from build123d import *

# Parameters (mm, degrees)
SKETCH1_R           = 10.75
SKETCH1_R_2         = 9.75
BOSS_EXTRUDE1_DEPTH = 1
SKETCH2_R           = 10.75
SKETCH2_R_2         = 9.75
BOSS_EXTRUDE2_DEPTH = 3.5
SKETCH3_R           = 10.75
BOSS_EXTRUDE3_DEPTH = 1.5
CUT_EXTRUDE1_DEPTH  = 1
BOSS_EXTRUDE4_DEPTH = 6
FILLET1_R           = 1.25
FILLET2_R           = 0.5


with BuildPart() as part:
    # Sketch1 → Boss-Extrude1 (new body)
    with BuildSketch(Plane(origin=(0, 0, 0), x_dir=(1, 0, 0), z_dir=(0, 1, 0))):
        with Locations(Location((0, 0, 0), (0, 0, 270))):
            Circle(SKETCH1_R)
        Circle(SKETCH1_R_2, mode=Mode.SUBTRACT)
        Circle(SKETCH1_R_2)
    extrude(amount=BOSS_EXTRUDE1_DEPTH)

    # Sketch2 → Boss-Extrude2 (add)
    with BuildSketch(Plane(origin=(0, 1, 0), x_dir=(1, 0, 0), z_dir=(0, 1, 0))):
        with Locations(Location((0, 0, 0), (0, 0, 270))):
            Circle(SKETCH2_R)
        with Locations(Location((0, 0, 0), (0, 0, 270))):
            Circle(SKETCH2_R_2, mode=Mode.SUBTRACT)
    extrude(amount=BOSS_EXTRUDE2_DEPTH)

    # Sketch3 → Boss-Extrude3 (add)
    with BuildSketch(Plane(origin=(0, 4.5, 0), x_dir=(1, 0, 0), z_dir=(0, 1, 0))):
        with Locations(Location((0, 0, 0), (0, 0, 270))):
            Circle(SKETCH3_R)
    extrude(amount=BOSS_EXTRUDE3_DEPTH)

    # Sketch4 → Cut-Extrude1 (cut)
    with BuildSketch(Plane(origin=(0, 6, 0), x_dir=(1, 0, 0), z_dir=(0, 1, 0))):
        Polygon((-9.25, -0.5), (-9.75, 0), (-9.25, 0.5), (-0.5, 0.5), (-0.5, 9.25), (0, 9.75), (0.5, 9.25), (0.5, 0.5), (9.25, 0.5), (9.75, 0), (9.25, -0.5), (0.5, -0.5), (0.5, -9.25), (0, -9.75), (-0.5, -9.25), (-0.5, -0.5), align=None)
        with BuildLine():
            ThreePointArc((-1.414213562, -0.5), (-1.5, 0), (-1.414213562, 0.5))
            Line((-1.414213562, 0.5), (-9.25, 0.5))
            Line((-9.25, 0.5), (-9.75, 0))
            Line((-9.75, 0), (-9.25, -0.5))
            Line((-9.25, -0.5), (-1.414213562, -0.5))
        make_face()
        with BuildLine():
            Line((9.25, 0.5), (1.414213562, 0.5))
            ThreePointArc((1.414213562, 0.5), (1.478397839, 0.253652968), (1.5, 0))
            ThreePointArc((1.5, 0), (1.478397839, -0.253652968), (1.414213562, -0.5))
            Line((1.414213562, -0.5), (9.25, -0.5))
            Line((9.25, -0.5), (9.75, 0))
            Line((9.75, 0), (9.25, 0.5))
        make_face()
        with BuildLine():
            Line((-0.5, 9.25), (-0.5, 1.414213562))
            ThreePointArc((-0.5, 1.414213562), (0, 1.5), (0.5, 1.414213562))
            Line((0.5, 1.414213562), (0.5, 9.25))
            Line((0.5, 9.25), (0, 9.75))
            Line((0, 9.75), (-0.5, 9.25))
        make_face()
        with BuildLine():
            ThreePointArc((0.5, -1.414213562), (0, -1.5), (-0.5, -1.414213562))
            Line((-0.5, -1.414213562), (-0.5, -9.25))
            Line((-0.5, -9.25), (0, -9.75))
            Line((0, -9.75), (0.5, -9.25))
            Line((0.5, -9.25), (0.5, -1.414213562))
        make_face()
        with BuildLine():
            Line((-0.5, -0.5), (-1.414213562, -0.5))
            ThreePointArc((-1.414213562, -0.5), (-1.060660172, -1.060660172), (-0.5, -1.414213562))
            Line((-0.5, -1.414213562), (-0.5, -0.5))
        make_face()
        with BuildLine():
            Line((-1.414213562, 0.5), (-0.5, 0.5))
            Line((-0.5, 0.5), (-0.5, 1.414213562))
            ThreePointArc((-0.5, 1.414213562), (-1.060660172, 1.060660172), (-1.414213562, 0.5))
        make_face()
        with BuildLine():
            ThreePointArc((1.414213562, 0.5), (1.060660172, 1.060660172), (0.5, 1.414213562))
            Line((0.5, 1.414213562), (0.5, 0.5))
            Line((0.5, 0.5), (1.414213562, 0.5))
        make_face()
        with BuildLine():
            Line((0.5, -0.5), (0.5, -1.414213562))
            ThreePointArc((0.5, -1.414213562), (1.060660172, -1.060660172), (1.414213562, -0.5))
            Line((1.414213562, -0.5), (0.5, -0.5))
        make_face()
    extrude(amount=-CUT_EXTRUDE1_DEPTH, mode=Mode.SUBTRACT)

    # Sketch6 → Boss-Extrude4 (add)
    with BuildSketch(Plane(origin=(0, 6, 0), x_dir=(1, 0, 0), z_dir=(0, 1, 0))):
        with BuildLine():
            Line((0.5, 1.414213562), (0.5, 3.464101615))
            ThreePointArc((0.5, 3.464101615), (2.474873734, 2.474873734), (3.464101615, 0.5))
            Line((3.464101615, 0.5), (1.414213562, 0.5))
            ThreePointArc((1.414213562, 0.5), (1.060660172, 1.060660172), (0.5, 1.414213562))
        make_face()
        with BuildLine():
            Line((0.5, -1.414213562), (0.5, -3.464101615))
            ThreePointArc((0.5, -3.464101615), (2.474873734, -2.474873734), (3.464101615, -0.5))
            Line((3.464101615, -0.5), (1.414213562, -0.5))
            ThreePointArc((1.414213562, -0.5), (1.060660172, -1.060660172), (0.5, -1.414213562))
        make_face()
        with BuildLine():
            Line((-1.414213562, -0.5), (-3.464101615, -0.5))
            ThreePointArc((-3.464101615, -0.5), (-2.474873734, -2.474873734), (-0.5, -3.464101615))
            Line((-0.5, -3.464101615), (-0.5, -1.414213562))
            ThreePointArc((-0.5, -1.414213562), (-1.060660172, -1.060660172), (-1.414213562, -0.5))
        make_face()
        with BuildLine():
            Line((-0.5, 1.414213562), (-0.5, 3.464101615))
            ThreePointArc((-0.5, 3.464101615), (-2.474873734, 2.474873734), (-3.464101615, 0.5))
            Line((-3.464101615, 0.5), (-1.414213562, 0.5))
            ThreePointArc((-1.414213562, 0.5), (-1.060660172, 1.060660172), (-0.5, 1.414213562))
        make_face()
    extrude(amount=BOSS_EXTRUDE4_DEPTH)

    # Fillet1
    fillet1_edges = [part.edges().sort_by_distance(p)[0] for p in [
        (-2.474873734, 6, 2.474873734),
        (-2.474873734, 6, -2.474873734),
        (2.474873734, 6, -2.474873734),
        (2.474873734, 6, 2.474873734),
    ]]
    fillet(fillet1_edges, radius=FILLET1_R)

    # Fillet2
    fillet2_edges = [part.edges().sort_by_distance(p)[0] for p in [
        (0, 6, -10.75),
        (0, 0, -10.75),
    ]]
    fillet(fillet2_edges, radius=FILLET2_R)


solid = part.part
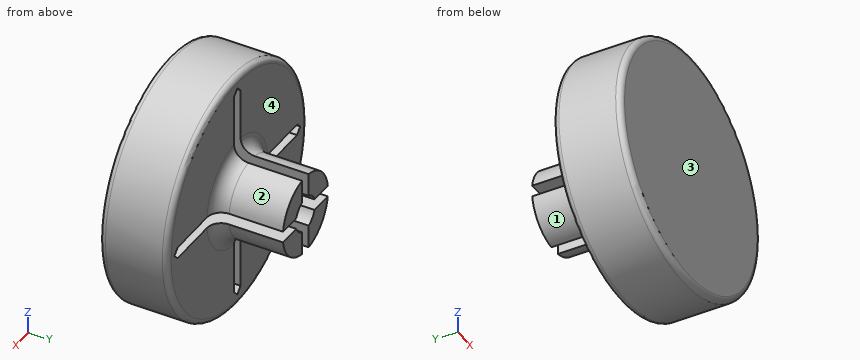
Design review of the part built by this model. Coordinates are the model's own, in mm. Face numbers are marked on the shaded views. A direction names the side the tool comes from. Round coordinates to 2 decimals unless told otherwise and drop trailing zeros. Write each loop counter-clockwise with the first axis right and the second up, starting at its lowest first coordinate (ties: lowest second). Pieces come first, ordered by that corner, then holes. Notation, with made-up numbers: (55.5, -10) -> (110.5, -10) arc R8 ccw to (110.5, 0) -> close; hole circle Ø1 at (6, 41). An arc over 180 degrees is marked (long way). One line per question, with ' | ' between items.
(1) Take a section at A-A, the plane y = 10.25. State the section outline as (x, z) points.
Result sheet:
outline: (-3.46, -0.5) arc R3.5 ccw to (-0.5, -3.46) -> (-0.5, -1.41) arc R1.5 cw to (-1.41, -0.5) -> close; (-3.46, 0.5) -> (-1.41, 0.5) arc R1.5 cw to (-0.5, 1.41) -> (-0.5, 3.46) arc R3.5 ccw to start; (0.5, -3.46) arc R3.5 ccw to (3.46, -0.5) -> (1.41, -0.5) arc R1.5 cw to (0.5, -1.41) -> close; (0.5, 1.41) arc R1.5 cw to (1.41, 0.5) -> (3.46, 0.5) arc R3.5 ccw to (0.5, 3.46) -> close
(2) Take a section at B-B, the plane y = 2.75. State the section outline as (x, z) points.
Result sheet:
outline: circle Ø21.5 at (0, 0); hole circle Ø19.5 at (0, 0)
(3) Wall thickness on line 1 (Y direction, x = -5.25, z = -6.25); line 2 (X direction, y = 1.9, z = 0); line 3 (X direction, y = 1.25, z = -2.5): over which ranges is each line inside the solid? List them lowest first. Write a range as [from, to].
Result sheet:
line 1: [0, 1], [4.5, 6] | line 2: [-10.75, -9.75], [9.75, 10.75] | line 3: [-10.46, -9.42], [9.42, 10.46]
(4) Machinability: for the marked faces 1, 2, 3 and 4, which of the approach directions +Z, -Z, +X, -X, +Y, -Y give a long, thin tool a straight path to every point of the face, cutting with its end or side? Answer none if there is none.
Result sheet:
face 1: -Z, -X, +Y | face 2: +Z, +X, +Y | face 3: +Z, -Z, +X, -X, -Y | face 4: +Y
(5) Insertion check: P1, Ø10, axis at x = 2, z = 1.5, coming from the -Y side; P2, Ø4, axis at x = -3.5, y = 6.5, coming from the -Z side; P3, Ø5.5, axis at x = -5.5, y = 7, coming from the -Z side; P4, Ø1.5, axis at y = 8, z = -1.5, coming from the +X side. Each pin has a flat end and moves straight along its axis. Give the tip position at first contact, or say it passes through.
Result sheet:
P1: y = 0 | P2: z = -10.61 | P3: z = -10.27 | P4: x = 3.42
